```python
from build123d import *

# Parameters (mm, degrees)
SKETCH_1_R      = 1.65
EXTRUDE_1_DEPTH = 1.45
SKETCH_5_W      = 1.05
SKETCH_5_H      = 1.756666667
FILLET_1_R      = 1.2
FILLET_3_R      = 0.15
FILLET_4_R      = 0.2
FILLET_5_R      = 0.3


with BuildPart() as part:
    # 草图1 → 凸台-拉伸1 (new, symmetric)
    with BuildSketch(Plane(origin=(0, 0, 0), x_dir=(1, 0, 0), z_dir=(0, 1, 0))):
        Polygon((4.041451884, 0), (2.020725942, 3.5), (-2.020725942, 3.5), (-4.041451884, 0), (-2.020725942, -3.5), (2.020725942, -3.5), align=None)
        with Locations(Location((0, 0, 0), (0, 0, 270))):
            Circle(SKETCH_1_R, mode=Mode.SUBTRACT)
    extrude(amount=EXTRUDE_1_DEPTH, both=True)

    # 草图4 → 旋转1 (revolve)
    with BuildSketch(Plane(origin=(0, 0, 0), x_dir=(0, 0, -1), z_dir=(1, 0, 0))):
        Polygon((-3.4, 1.45), (-3.4, 3.55), (-2, 3.55), (-2, 3.216666667), (-2.5, 3.216666667), (-2.5, 1.45), align=None)
    revolve(axis=Axis((0, 2.804536462, 0), (0, -1, 0)))

    # 草图5 → 旋转2 (revolve)
    with BuildSketch(Plane(origin=(0, 0, 0), x_dir=(0, 0, -1), z_dir=(1, 0, 0))):
        with Locations((-1.975, 2.328333334)):
            Rectangle(SKETCH_5_W, SKETCH_5_H)
    revolve(axis=Axis((0, 2.51357275, 0), (0, -1, 0)))

    # 圆角1
    fillet_1_edges = [part.edges().sort_by_distance(p)[0] for p in [
        (0, 3.55, -3.4),
    ]]
    fillet(fillet_1_edges, radius=FILLET_1_R)

    # 圆角3
    fillet_3_edges = [part.edges().sort_by_distance(p)[0] for p in [
        (0, 3.55, -2),
    ]]
    fillet(fillet_3_edges, radius=FILLET_3_R)

    # 草图6 → 切除-旋转1 (revolve, cut)
    with BuildSketch(Plane(origin=(0, 0, 0), x_dir=(0, 0, -1), z_dir=(1, 0, 0)), mode=Mode.PRIVATE) as cut_revolve_1_sk:
        Polygon((3.4, 1.45), (5.824871131, 1.45), (5.824871131, 0.05), align=None)
        Polygon((5.824871131, -0.05), (3.4, -1.45), (5.824871131, -1.45), align=None)
    revolve(cut_revolve_1_sk.sketch.rotate(Axis((0, 2.537572, 0), (0, -1, 0)), 30.000000005), axis=Axis((0, 2.537572, 0), (0, -1, 0)), mode=Mode.SUBTRACT)

    # 圆角4
    fillet_4_edges = [part.edges().sort_by_distance(p)[0] for p in [
        (3.284147809, 1.45, 0.879984753),
    ]]
    fillet(fillet_4_edges, radius=FILLET_4_R - 0.0001)  # a hair under: the kernel refuses the full size

    # 圆角5
    fillet_5_edges = [part.edges().sort_by_distance(p)[0] for p in [
        (-1.7, -1.45, 2.944486373),
    ]]
    fillet(fillet_5_edges, radius=FILLET_5_R)


solid = part.part
```
Geometry check sheet. Reference: the model listing, model coordinates, mm. A direction names the side the tool comes from. Round coordinates to 2 decimals unless told otherwise and drop trailing zeros. Loops run counter-clockwise (first coordinate to the right, second up) from the corner with the lowest first, then second, coordinate; pieces in that order, holes last. Notation, with made-up numbers: (17, 43.5) - (58, 43.5) arc R6 ccw to (58, 47.5) - close; hole circle Ø8 at (-31, -24). An arc over 180 degrees is marked (long way). Write item = value, one per line. Start each with the question number.
1. Thickness scan on line 1 (X direction, y = 2.1, z = 0); line 2 (X direction, y = -0.35, z = 0.25); line 3 (Z direction, x = 0, y = 3.25). Record the ranges inside material, lowest first.
2. Section check A-A on y = 2.75. Enter the section's corners in (x, z).
3. Mould release check, pull along X, two halves, no side actions. Record for faces 6 (the face through (0, 0, 3.5)), 7 (the face through (3.045, 0.019, -1.726)), 8 (the face through (-3, 0, -1.8)), 9 (the face through (-1.22, 2.34, 0.78)): released by +X, released by -X, zero draft, split by the parting line, or undercut.
4. Depth check by flat-ended pin: pin 1 (1.6 mm diameter, centred on x = 0.5, z = -0.5, fed in from -Y); pin 2 (4 mm diameter, centred on x = 0, z = 0, fed in from -Y); pin 3 (1.5 mm diameter, centred on y = -1, z = 1, fed in from +X). Enter the tip coordinate at first touch or a pass-through.
5. Set-up check for faces 1 (the face through (-2.298, 1.963, -2.506)), 2 (the face through (0, 0, -3.5)), 3 (the face through (-1, -0.02, -1.31)), 4 (the face through (0, 3.207, 1.6)), 5 (the face through (3, 0, 1.8)): record each of +Z, -Z, +X, -X, +Y, -Y from which the full face is reachable in a straight line by a thin tool's end or side.
Working result:
q1.line_1 = -3.4 to -1.45, 1.45 to 3.4
q1.line_2 = -3.9 to -1.63, 1.63 to 3.9
q1.line_3 = -2.99 to -2, 2 to 2.99
q2.outline = circle Ø6.66 at (0, 0); hole circle Ø2.9 at (0, 0)
q3.face_6 = zero draft
q3.face_7 = released by +X
q3.face_8 = released by -X
q3.face_9 = undercut
q4.pin_1 = 1.45
q4.pin_2 = -1.45
q4.pin_3 = 3.9
q5.face_1 = +Y
q5.face_2 = -Z, +X, -X, +Y, -Y
q5.face_3 = -Y
q5.face_4 = none
q5.face_5 = +Z, +X, +Y, -Y
